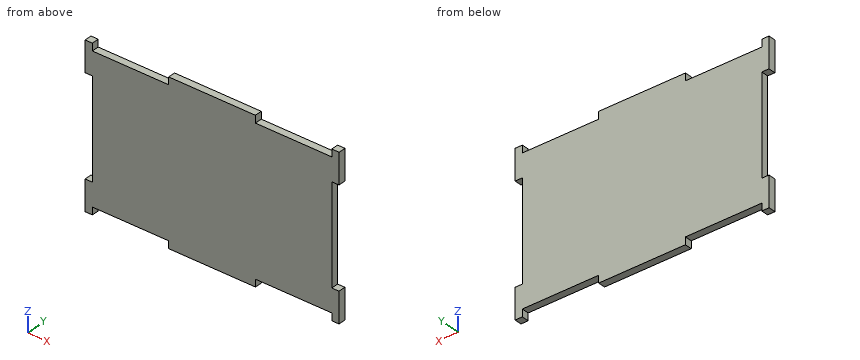
```python
from build123d import *

# Parameters (mm, degrees)
SKETCH1_W           = 38
SKETCH1_H           = 3.175
BOSS_EXTRUDE1_DEPTH = 3.175


with BuildPart() as part:
    # Sketch1 → Boss-Extrude1 (new body)
    with BuildSketch(Plane(origin=(0, 0, 0), x_dir=(1, 0, 0), z_dir=(0, 1, 0))):
        Polygon((0, 13.275), (0, 0), (3.175, 0), (3.175, 3.175), (36.675, 3.175), (74.675, 3.175), (108.175, 3.175), (108.175, 0), (111.35, 0), (111.35, 13.275), (108.175, 13.275), (108.175, 56.275), (111.35, 56.275), (111.35, 69.55), (108.175, 69.55), (108.175, 66.375), (74.675, 66.375), (36.675, 66.375), (3.175, 66.375), (3.175, 69.55), (0, 69.55), (0, 56.275), (3.175, 56.275), (3.175, 13.275), align=None)
        with Locations((55.675, 67.9625)):
            Rectangle(SKETCH1_W, SKETCH1_H)
        with Locations((55.675, 1.5875)):
            Rectangle(SKETCH1_W, SKETCH1_H)
    extrude(amount=BOSS_EXTRUDE1_DEPTH)


solid = part.part
```
CAD build for the part. Positions are in the model's coordinates, mm. Round coordinates to 2 decimals unless told otherwise and drop trailing zeros. Order: outer loops, then holes, each group sorted by start corner. A loop starts at its lowest first (then second) coordinate and runs counter-clockwise, first axis right, second up.
Item 1: Probe line 1 along X through (y, z) = (0.95, -2.5) (3 decimals); line 2 along Z through (x, y) = (25, 2.15) (3 decimals); line 3 along X through (y, z) = (0.8, -31) (3 decimals). List the from-to ranges inside material, lowest first.
Item 2: Saw through at B-B on z = -30.5. Write the cut outline in (x, y) (3 decimals).
Item 3: Pin check, flat tips, straight feed: pin 1 (1 mm diameter, centred on x = 15, y = 1, fed in from -Z) (3 decimals); pin 2 (1.6 mm diameter, centred on y = 1, z = -37, fed in from +X) (3 decimals); pin 3 (1 mm diameter, centred on x = 86.5, y = 2, fed in from +Z) (3 decimals). Stop position of each tip, or through.
Item 4: Saw through at C-C on x = 82.5. Write the cut outline in (y, z) (3 decimals), then the cut area to 3 significant figures.
Item 5: Saw through at A-A on y = 1.4. Write the cut outline in (x, z) (3 decimals).
Reported:
1. line 1: x = 0 to 3.175, 36.675 to 74.675, 108.175 to 111.35
1. line 2: z = -66.375 to -3.175
1. line 3: x = 3.175 to 108.175
2. outline: (3.175, 0) - (108.175, 0) - (108.175, 3.175) - (3.175, 3.175) - close
3. pin 1: stops at z = -66.375
3. pin 2: stops at x = 108.175
3. pin 3: stops at z = -3.175
4. outline: (0, -66.375) - (3.175, -66.375) - (3.175, -3.175) - (0, -3.175) - close
4. area: 201 mm2
5. outline: (0, -69.55) - (3.175, -69.55) - (3.175, -66.375) - (36.675, -66.375) - (36.675, -69.55) - (74.675, -69.55) - (74.675, -66.375) - (108.175, -66.375) - (108.175, -69.55) - (111.35, -69.55) - (111.35, -56.275) - (108.175, -56.275) - (108.175, -13.275) - (111.35, -13.275) - (111.35, 0) - (108.175, 0) - (108.175, -3.175) - (74.675, -3.175) - (74.675, 0) - (36.675, 0) - (36.675, -3.175) - (3.175, -3.175) - (3.175, 0) - (0, 0) - (0, -13.275) - (3.175, -13.275) - (3.175, -56.275) - (0, -56.275) - close
